Geometry: final body of the model. Coordinates: model frame, mm. A direction names the side the tool comes from. Give positions to 0.01 mm unless a question says otherwise; leave off trailing zeros. Loops run counter-clockwise (first coordinate to the right, second up) from the corner with the lowest first, then second, coordinate; pieces in that order, holes last. Notation, with made-up numbers: (-34, -20) -> (2, -20) arc R22 cw to (2, -11) -> close; hole circle Ø8 at (47.5, -32). An arc over 180 degrees is marked (long way). One line per item, written item: value. Start each with the question number.
from build123d import *

# Parameters (mm, degrees)
SKETCH1_R           = 25
BOSS_EXTRUDE2_DEPTH = 75
SKETCH2_R           = 12.5
SKETCH2_W           = 1
SKETCH2_H           = 20
BOSS_EXTRUDE3_DEPTH = 30
FILLET2_R           = 2


with BuildPart() as part:
    # Sketch1 → Boss-Extrude2 (new body, symmetric)
    with BuildSketch(Plane.XY):
        Circle(SKETCH1_R)
    extrude(amount=BOSS_EXTRUDE2_DEPTH, both=True)

    # Sketch2 → Boss-Extrude3 (add)
    with BuildSketch(Plane.XY.offset(75)):
        Circle(SKETCH2_R)
        Rectangle(SKETCH2_W, SKETCH2_H, mode=Mode.SUBTRACT)
    boss_extrude3 = extrude(amount=BOSS_EXTRUDE3_DEPTH)

    # Mirror1: Boss-Extrude3 across plane
    add(boss_extrude3.mirror(Plane.XY))

    # Fillet2
    fillet2_edges = [part.edges().sort_by_distance(p)[0] for p in [
        (-25, 0, -75),
        (-25, 0, 75),
    ]]
    fillet(fillet2_edges, radius=FILLET2_R)


solid = part.part
Item 1: Mould query, pull axis X, two halves, no side actions, for faces 1 (the face through (11.923, 3.755, -89.79)), 2 (the face through (-0.5, 0, 90)), 3 (the face through (10, -10, 75)). Classes: pulls with the +X half, pulls with the -X half, needs draft (parallel to the pull), parting line crosses it, or undercut.
Item 2: Pin query (flat end, axial travel): pin 1 (8 mm diameter, centred on y = 16, z = 65, fed in from -X); pin 2 (6 mm diameter, centred on y = 0, z = -84, fed in from +X); pin 3 (1 mm diameter, centred on x = 14.5, y = 5.5, fed in from -Z); pin 4 (23 mm diameter, centred on x = -9.5, y = 10, fed in from +Z). Return the tip coordinate at first contact, or that it passes through.
Item 3: Ray query, line 1 along Y through (x, z) = (-0.5, -61) (3 decimals); line 2 along Z through (x, y) = (-15, -12); line 3 along Y through (x, z) = (-18, -0.5). Return the intervals inside material, ascending. Write a range as [from, to].
Item 4: Section A-A, the plane y = 0. Output: boundary loops of the cut face in (x, z), then the cut area to 3 significant figures.
Item 5: Section B-B, the plane z = -43. Output: boundary loops of the cut face in (x, y).
Item 6: Access query for faces 4 (the face through (0.5, 0, -90)), 5 (the face through (0.5, 0, 90)), 6 (the face through (23.846, 7.509, 1.022)). Directions: +Z, -Z, +X, -X, +Y, -Y. A direction counts if a zero-diameter tool reaches every point of the face in a straight line with its end or side. Return the directions, or none.
Geometry check:
1. face 1: parting line crosses it
1. face 2: undercut
1. face 3: needs draft
2. pin 1: stops at x = -21.93
2. pin 2: stops at x = 12.5
2. pin 3: stops at z = -75
2. pin 4: stops at z = 105
3. line 1: y = [-24.995, 24.995]
3. line 2: z = [-75, 75]
3. line 3: y = [-17.35, 17.35]
4. outline: (-25, -73) arc R2 ccw to (-23, -75) -> (-12.5, -75) -> (-12.5, -105) -> (-0.5, -105) -> (-0.5, -75) -> (0.5, -75) -> (0.5, -105) -> (12.5, -105) -> (12.5, -75) -> (23, -75) arc R2 ccw to (25, -73) -> (25, 73) arc R2 ccw to (23, 75) -> (12.5, 75) -> (12.5, 105) -> (0.5, 105) -> (0.5, 75) -> (-0.5, 75) -> (-0.5, 105) -> (-12.5, 105) -> (-12.5, 75) -> (-23, 75) arc R2 ccw to (-25, 73) -> close
4. area: 8,940 mm2
5. outline: circle Ø50 at (0, 0)
6. face 4: -Z
6. face 5: +Z
6. face 6: +Z, -Z
